The model under review builds one solid part; all positions refer to its coordinate system, in mm. Give positions to 0.01 mm unless a question says otherwise; leave off trailing zeros. Loops run counter-clockwise (first coordinate to the right, second up) from the corner with the lowest first, then second, coordinate; pieces in that order, holes last. Notation, with made-up numbers: (9.5, 6) - (40.5, 6) arc R19 ccw to (40.5, 12) - close; hole circle Ø7 at (72, -2). An arc over 180 degrees is marked (long way). Return JSON: item names as keys, results as strings. Group by question number.
```python
from build123d import *

# Parameters (mm, degrees)
SKETCH1_W           = 78.5
SKETCH1_H           = 78.5
BOSS_EXTRUDE1_DEPTH = 3.5
FILLET1_R           = 10
SKETCH2_R           = 2
CUT_EXTRUDE1_DEPTH  = 56.947520052
SKETCH3_R           = 18.5
CUT_EXTRUDE2_DEPTH  = 56.947520052
SKETCH4_R           = 2
CUT_EXTRUDE3_DEPTH  = 56.947520052


with BuildPart() as part:
    # Sketch1 → Boss-Extrude1 (new, symmetric)
    with BuildSketch(Plane.XY):
        Rectangle(SKETCH1_W, SKETCH1_H)
    extrude(amount=BOSS_EXTRUDE1_DEPTH, both=True)

    # Fillet1
    fillet1_edges = [part.edges().sort_by_distance(p)[0] for p in [
        (39.25, -39.25, 0),
        (-39.25, -39.25, 0),
        (-39.25, 39.25, 0),
        (39.25, 39.25, 0),
    ]]
    fillet(fillet1_edges, radius=FILLET1_R)

    # Sketch2 → Cut-Extrude1 (cut, through all)
    with BuildSketch(Plane.XY.offset(3.5)):
        with Locations((-31.371320344, 31.371320344)):
            Circle(SKETCH2_R)
        with Locations(Location((-31.371320344, -31.371320344, 0), (0, 0, 180))):
            Circle(SKETCH2_R)
        with Locations(Location((31.371320344, 31.371320344, 0), (0, 0, 180))):
            Circle(SKETCH2_R)
        with Locations((31.371320344, -31.371320344)):
            Circle(SKETCH2_R)
    extrude(amount=-CUT_EXTRUDE1_DEPTH, mode=Mode.SUBTRACT)

    # Sketch3 → Cut-Extrude2 (cut, through all)
    with BuildSketch(Plane.XY.offset(3.5)):
        Circle(SKETCH3_R)
    extrude(amount=-CUT_EXTRUDE2_DEPTH, mode=Mode.SUBTRACT)

    # Sketch4 → Cut-Extrude3 (cut, through all)
    with BuildSketch(Plane.XY.offset(3.5)):
        with Locations((0, 33.333013665)):
            Circle(SKETCH4_R)
        with Locations((-33.333013665, 0)):
            Circle(SKETCH4_R)
        with Locations((0, -33.333013665)):
            Circle(SKETCH4_R)
        with Locations((33.333013665, 0)):
            Circle(SKETCH4_R)
    extrude(amount=-CUT_EXTRUDE3_DEPTH, mode=Mode.SUBTRACT)


solid = part.part
```
1) Draft analysis for pull direction Y (two halves, no side actions). For faces 1 (the face through (31.63, 29.39, 0.05)), 2 (the face through (-36.4, 36.24, -0.05)), 3 (the face through (-36.4, -36.24, 0.05)), 4 (the face through (-0.26, 35.316, 0.049)), state which applies: +Y half, -Y half, draft (parallel to the pull), parting line (faces both ways), or undercut.
2) We need section C-C, the plane z = 0.75. Count the separate pieces of the cut face and the enclosed holes in it, plus the area to 3 significant figures.
3) We need section A-A, the plane y = 0. Write out the cut boundary in (x, z), plus the area to 4 significant figures.
4) For pin 1 Ø6.5 at (x, y) = (31.37, 31.37) entering from -Z, flat-tipped, find the tip position at first contact; note if it passes through.
5) To check wall thickness, follow line 1 (Y direction, x = 0, z = -1); line 2 (Y direction, x = -30.5, z = 3.25); line 3 (X direction, y = -32.5, z = -0.75). State the ranges of each line that lie inside material, in increasing order.
6) We need section D-D, the plane y = 10.5. Write out the cut boundary in (x, z), plus the area to 3 significant figures.
Findings:
{
 "1": {"face 1": "undercut", "face 2": "+Y half", "face 3": "-Y half", "face 4": "undercut"},
 "2": {"separate pieces": "1", "enclosed holes": "9", "area": "4,900 mm^2"},
 "3": {"outline": "(-39.25, -3.5) - (-35.33, -3.5) - (-35.33, 3.5) - (-39.25, 3.5) - close; (-31.33, -3.5) - (-18.5, -3.5) - (-18.5, 3.5) - (-31.33, 3.5) - close; (18.5, -3.5) - (31.33, -3.5) - (31.33, 3.5) - (18.5, 3.5) - close; (35.33, -3.5) - (39.25, -3.5) - (39.25, 3.5) - (35.33, 3.5) - close", "area": "234.5 mm^2"},
 "4": {"pin 1": "stops at z = -3.5"},
 "5": {"line 1": "y = -39.25 to -35.33, -31.33 to -18.5, 18.5 to 31.33, 35.33 to 39.25", "line 2": "y = -39.17 to -33.17, -29.57 to 29.57, 33.17 to 39.17", "line 3": "x = -38.71 to -33.02, -29.72 to -1.82, 1.82 to 29.72, 33.02 to 38.71"},
 "6": {"outline": "(-39.25, -3.5) - (-15.23, -3.5) - (-15.23, 3.5) - (-39.25, 3.5) - close; (15.23, -3.5) - (39.25, -3.5) - (39.25, 3.5) - (15.23, 3.5) - close", "area": "336 mm^2"}
}
